The listing builds one solid part. Answer for the finished solid, in the listing's coordinates (mm). Face numbers are marked on the shaded views. A direction names the side the tool comes from. Give positions to 0.01 mm unless a question says otherwise; leave off trailing zeros. Order: outer loops, then holes, each group sorted by start corner. A loop starts at its lowest first (then second) coordinate and runs counter-clockwise, first axis right, second up. Notation, with made-up numbers: (88.5, -23) - (116.5, -23) arc R21 cw to (116.5, 10) - close; hole circle Ø8 at (44.5, -18). An arc over 180 degrees is marked (long way). Answer as CSV lines item,"result". Start each with the question number.
1. Which of the six approach directions +Z, -Z, +X, -X, +Y, -Y give full straight-line access (tool end or side, diameter ignored) to the marked faces 1, 2, 3 and 4?
2. Section B-B on y = 0 is taken. Give the vertices of the cut face in (x, z).
3. Section D-D on z = 14 is taken. Give the vertices of the cut face in (x, y).
4. Section A-A on x = -2.75 is taken. Count the separate pieces of the cut face and the enclosed holes in it, and give its area (3 significant figures).
5. Flat-ended cylindrical pins translate along their axes: pin 1 (1.6 mm diameter, centred on x = -7, z = 26, fed in from -Y); pin 2 (1 mm diameter, centred on x = -6, z = 28.5, fed in from +Y); pin 3 (4 mm diameter, centred on x = 1, y = 1, fed in from +Z). Find the tip coordinate at first contact, or state that the pin passes through.
6. Consider line 1 along X through (y, z) = (-7, 27); line 2 along Z through (x, y) = (-7.8, 0); line 3 along Y through (x, z) = (-2, 19). Determine where each line is inside the solid, lowest interval first. Write a range as [from, to].
7. Determine the mould class of the marked faces 5, 6, 7 and 8 for opening direction X: +X half, -X half, draft (parallel to the pull), parting line (faces both ways), or undercut.
from build123d import *

# Parameters (mm, degrees)
SKETCH_W        = 19
SKETCH_H        = 35
PAD_DEPTH       = 2
SKETCH001_W     = 19
SKETCH001_H     = 35
SKETCH001_W_2   = 13
SKETCH001_H_2   = 29
PAD001_DEPTH    = 32
SKETCH002_W     = 12.5
SKETCH002_H     = 8
POCKET_DEPTH    = 3
FILLET_R        = 1
SKETCH003_W     = 13
SKETCH003_H     = 12
POCKET001_DEPTH = 2
SKETCH004_W     = 5
SKETCH004_H     = 8.323044
POCKET002_DEPTH = 1
SKETCH005_W     = 5
SKETCH005_H     = 12
POCKET003_DEPTH = 3
CHAMFER_SIZE    = 2.999
FILLET001_R     = 1
FILLET002_R     = 1
FILLET003_R     = 1
FILLET004_R     = 1
FILLET005_R     = 1
FILLET006_R     = 1
FILLET007_R     = 1
FILLET008_R     = 1
FILLET009_R     = 1
CHAMFER001_SIZE = 2.999
SKETCH006_R     = 1.5
POCKET004_DEPTH = 5


with BuildPart() as part:
    # Sketch → Pad (new body)
    with BuildSketch(Plane.XY):
        Rectangle(SKETCH_W, SKETCH_H)
    extrude(amount=PAD_DEPTH)

    # Sketch001 (on Face6 of Pad) → Pad001 (join)
    with BuildSketch(Plane.XY.offset(2)):
        Rectangle(SKETCH001_W, SKETCH001_H)
        Rectangle(SKETCH001_W_2, SKETCH001_H_2, mode=Mode.SUBTRACT)
    extrude(amount=PAD001_DEPTH)

    # Sketch002 (on Face10 of Pad001) → Pocket (cut)
    with BuildSketch(Plane.XZ.offset(17.5)):
        with Locations((-3.25, 26)):
            Rectangle(SKETCH002_W, SKETCH002_H)
    extrude(amount=-POCKET_DEPTH, mode=Mode.SUBTRACT)

    # Fillet
    fillet_edges = [part.edges().sort_by_distance(p)[0] for p in [
        (3, -17.5, 26),
        (-3.25, -17.5, 30),
        (-3.25, -17.5, 22),
    ]]
    fillet(fillet_edges, radius=FILLET_R)

    # Sketch003 (on Face2 of Fillet) → Pocket001 (cut)
    with BuildSketch(Plane.XZ.offset(17.5)):
        with Locations((-3, 11.5)):
            Rectangle(SKETCH003_W, SKETCH003_H)
    extrude(amount=-POCKET001_DEPTH, mode=Mode.SUBTRACT)

    # Sketch004 (on Face9 of Pocket001) → Pocket002 (cut)
    with BuildSketch(Plane.XZ.offset(15.5)):
        with Locations((-0.838478, 11.5)):
            Rectangle(SKETCH004_W, SKETCH004_H)
    extrude(amount=-POCKET002_DEPTH, mode=Mode.SUBTRACT)

    # Sketch005 (on Face12 of Pocket002) → Pocket003 (cut)
    with BuildSketch(Plane(origin=(0, 17.5, 0), x_dir=(-1, 0, 0), z_dir=(0, 1, 0))):
        with Locations((2, 28)):
            Rectangle(SKETCH005_W, SKETCH005_H)
    extrude(amount=-POCKET003_DEPTH, mode=Mode.SUBTRACT)

    # Chamfer
    chamfer_edges = [part.edges().sort_by_distance(p)[0] for p in [
        (0.5, 17.5, 28),
        (-4.5, 17.5, 28),
    ]]
    chamfer(chamfer_edges, length=CHAMFER_SIZE)

    # Fillet001
    fillet001_edges = [part.edges().sort_by_distance(p)[0] for p in [
        (-3, -17.5, 17.5),
        (3.5, -17.5, 11.5),
        (-3, -17.5, 5.5),
    ]]
    fillet(fillet001_edges, radius=FILLET001_R)

    # Fillet002
    fillet002_edges = [part.edges().sort_by_distance(p)[0] for p in [
        (0, -17.5, 0),
    ]]
    fillet(fillet002_edges, radius=FILLET002_R)

    # Fillet003
    fillet003_edges = [part.edges().sort_by_distance(p)[0] for p in [
        (9.5, 0.5, 0),
    ]]
    fillet(fillet003_edges, radius=FILLET003_R)

    # Fillet004
    fillet004_edges = [part.edges().sort_by_distance(p)[0] for p in [
        (-0.5, 17.5, 0),
    ]]
    fillet(fillet004_edges, radius=FILLET004_R)

    # Fillet005
    fillet005_edges = [part.edges().sort_by_distance(p)[0] for p in [
        (-9.5, 0, 0),
    ]]
    fillet(fillet005_edges, radius=FILLET005_R)

    # Fillet006
    fillet006_edges = [part.edges().sort_by_distance(p)[0] for p in [
        (-0.5, -17.5, 34),
    ]]
    fillet(fillet006_edges, radius=FILLET006_R)

    # Fillet007
    fillet007_edges = [part.edges().sort_by_distance(p)[0] for p in [
        (-9.5, 0, 34),
    ]]
    fillet(fillet007_edges, radius=FILLET007_R)

    # Fillet008
    fillet008_edges = [part.edges().sort_by_distance(p)[0] for p in [
        (-9.5, -15.5, 11.5),
    ]]
    fillet(fillet008_edges, radius=FILLET008_R)

    # Fillet009
    fillet009_edges = [part.edges().sort_by_distance(p)[0] for p in [
        (-9.5, -14.5, 26),
    ]]
    fillet(fillet009_edges, radius=FILLET009_R)

    # Chamfer001
    chamfer001_edges = [part.edges().sort_by_distance(p)[0] for p in [
        (-2, 17.5, 22),
    ]]
    chamfer(chamfer001_edges, length=CHAMFER001_SIZE)

    # Sketch006 (on Face16 of Chamfer001) → Pocket004 (cut)
    with BuildSketch(Plane(origin=(-9.5, 0, 0), x_dir=(0, -1, 0), z_dir=(-1, 0, 0))):
        with Locations((0, 31)):
            Circle(SKETCH006_R)
    extrude(amount=-POCKET004_DEPTH, mode=Mode.SUBTRACT)


solid = part.part
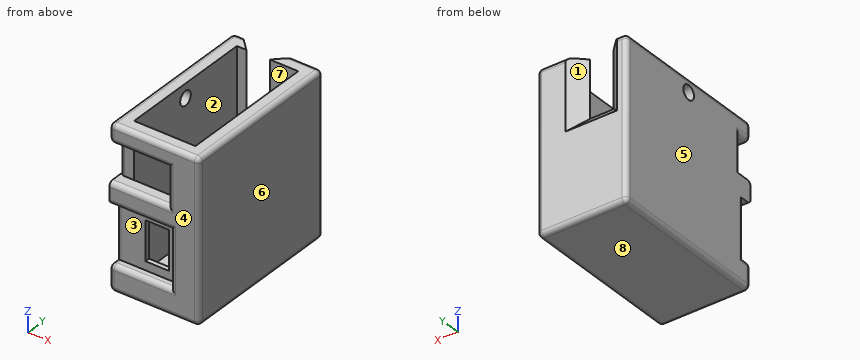
Checks:
1,face 1,"+Z, +Y"
1,face 2,"+Z"
1,face 3,"-X, -Y"
1,face 4,"+Z, -Z, +X, -X, -Y"
2,outline,"(-9.5, 1) arc R1 ccw to (-8.5, 0) - (8.5, 0) arc R1 ccw to (9.5, 1) - (9.5, 33) arc R1 ccw to (8.5, 34) - (6.5, 34) - (6.5, 2) - (-6.5, 2) - (-6.5, 29.5) - (-9.5, 29.5) - close; (-9.5, 32.5) - (-6.5, 32.5) - (-6.5, 34) - (-8.5, 34) arc R1 ccw to (-9.5, 33) - close"
3,outline,"(-9.5, -14.5) arc R1 ccw to (-8.5, -15.5) - (-3.34, -15.5) - (-3.34, -14.5) - (-6.5, -14.5) - (-6.5, 14.5) - (6.5, 14.5) - (6.5, -14.5) - (1.66, -14.5) - (1.66, -15.5) - (3.5, -15.5) - (3.5, -16.5) arc R1 ccw to (4.5, -17.5) - (8.5, -17.5) arc R1 ccw to (9.5, -16.5) - (9.5, 16.5) arc R1 ccw to (8.5, 17.5) - (-8.5, 17.5) arc R1 ccw to (-9.5, 16.5) - close"
4,separate pieces,"3"
4,enclosed holes,"0"
4,area,"164 mm²"
5,pin 1,"stops at y = -14.5"
5,pin 2,"stops at y = 16.5"
5,pin 3,"stops at z = 2"
6,line 1,"x = [-9.5, -6.5], [6.5, 9.5]"
6,line 2,"z = [0, 29.5], [32.5, 34]"
6,line 3,"y = [-17.5, -14.5], [14.5, 17.5]"
7,face 5,"-X half"
7,face 6,"+X half"
7,face 7,"undercut"
7,face 8,"draft"
